Design review of the part shown in the three views and the two pictorial views. Dimensions are in mm from the part's minimum x, y and z. A direction names the side the tool comes from. Give positions to 0.01 mm unless a question says otherwise; leave off trailing zeros. Loops run counter-clockwise (first coordinate to the right, second up) from the corner with the lowest first, then second, coordinate; pieces in that order, holes last.
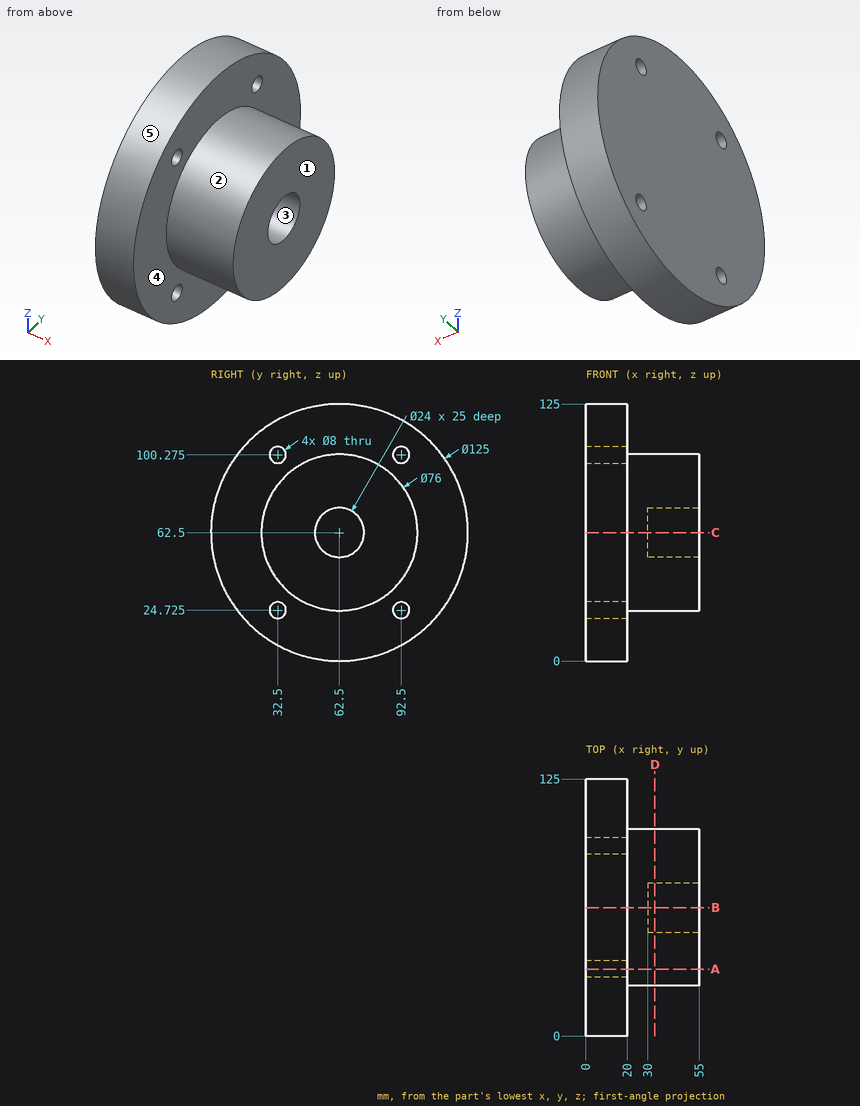
Q1. Mouldability with a two-part tool opening along Z and no side actions: class the marked faces 1, 2 and 3 as +Z half, -Z half, draft (parallel to the pull), parting line (faces both ways), or undercut.
Answers:
face 1: draft
face 2: parting line
face 3: undercut
Q2. Consider section A-A on y = 32.5. Give the boundary of the cut face in (x, z) (3 decimals).
Answers:
outline: (0, 7.671) - (20, 7.671) - (20, 20.725) - (0, 20.725) - close; (0, 28.725) - (20, 28.725) - (20, 39.176) - (55, 39.176) - (55, 85.824) - (20, 85.824) - (20, 96.275) - (0, 96.275) - close; (0, 104.275) - (20, 104.275) - (20, 117.329) - (0, 117.329) - close
Q3. Consider section B-B on y = 62.5. Give the boundary of the cut face in (x, z), plus the area to 3 significant figures.
Answers:
outline: (0, 0) - (20, 0) - (20, 24.5) - (55, 24.5) - (55, 50.5) - (30, 50.5) - (30, 74.5) - (55, 74.5) - (55, 100.5) - (20, 100.5) - (20, 125) - (0, 125) - close
area: 4,560 mm2
Q4. Machinability: for the marked faces 4 and 5, which of the approach directions +Z, -Z, +X, -X, +Y, -Y give a long, thin tool a straight path to every point of the face, cutting with its end or side? Answer none if there is none.
Answers:
face 4: +X
face 5: +X, -X
Q5. For probe 1 along Y at (x, z) = (10, 22.5); probe 2 along Y at (x, z) = (42, 62); probe 3 along Z at (x, y) = (5, 32), list the stretches that pass through material, from the lowest coordinate up.
Answers:
probe 1: y = 14.48 to 29.18, 35.82 to 89.18, 95.82 to 110.52
probe 2: y = 24.5 to 50.51, 74.49 to 100.5
probe 3: z = 7.95 to 20.76, 28.69 to 96.31, 104.24 to 117.05
Q6. For pin 1 Ø1.5 at (x, z) = (25.5, 30.5) entering from -Y; pin 2 Ø4 at (y, z) = (67.5, 20.5) entering from +X; pin 3 Ø4 at (x, y) = (47, 35) entering from -Z, all flat-tipped, find the tip position at first contact; note any pin that passes through.
Answers:
pin 1: stops at y = 40.88
pin 2: stops at x = 20
pin 3: stops at z = 34.33
Q7. Consider section D-D on x = 33.5. Give the boundary of the cut face in (y, z).
Answers:
outline: circle Ø76 at (62.5, 62.5); hole circle Ø24 at (62.5, 62.5)
